Design review of the part built by this model. Coordinates are the model's own, in mm. Give positions to 0.01 mm unless a question says otherwise; leave off trailing zeros. Write each loop counter-clockwise with the first axis right and the second up, starting at its lowest first coordinate (ties: lowest second). Pieces come first, ordered by that corner, then holes. Notation, with made-up numbers: (12.25, 34.25) -> (51.25, 34.25) arc R23 ccw to (51.25, 60.25) -> close; hole circle Ø9 at (14, 27). An arc over 180 degrees is marked (long way). Use CSV: the item, a comma, the result in double quotes.
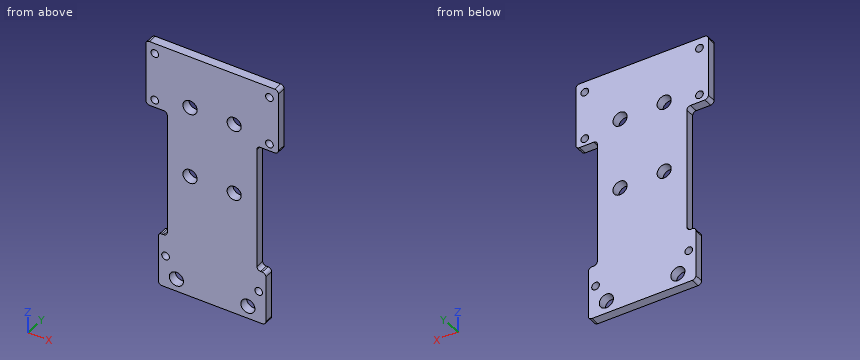
Autodesk Inventor part; units mm, degrees
ref_plane "YZ Plane" through (0, 0, 0) normal (1, 0, 0) x (0, 1, 0)
ref_plane "XZ Plane" through (0, 0, 0) normal (0, 1, 0) x (-1, 0, 0)
ref_plane "XY Plane" through (0, 0, 0) normal (0, 0, 1) x (1, 0, 0)
sketch "Sketch2" plane through (0, 0, 0) normal (0, 1, 0) x (-1, 0, 0)
  line L0 (35, 0) -> (-35, 0)
  line L1 (-37, -2) -> (-37, -35)
  line L2 (-35, -37) -> (-27, -37)
  line L3 (-25, -39) -> (-25, -107)
  line L4 (-27, -109) -> (-28, -109)
  line L5 (-30, -111) -> (-30, -137)
  line L6 (-28, -139) -> (28, -139)
  line L7 (30, -137) -> (30, -111)
  line L8 (28, -109) -> (27, -109)
  line L9 (25, -107) -> (25, -39)
  line L10 (27, -37) -> (35, -37)
  line L11 (37, -35) -> (37, -2)
  circle A0 centre (19.95, -132) radius 3.95
  circle A1 centre (-19.95, -132) radius 3.95
  circle A2 centre (26, -121) radius 2.15
  circle A3 centre (-26, -121) radius 2.15
  circle A4 centre (12.319, -69.4) radius 3.95
  circle A5 centre (-12.321, -69.4) radius 3.95
  circle A6 centre (12.319, -29.4) radius 3.95
  circle A7 centre (-12.319, -29.4) radius 3.95
  circle A8 centre (32, -32.8) radius 2.15
  circle A9 centre (32, -5.8) radius 2.15
  circle A10 centre (-32, -33) radius 2.15
  circle A11 centre (-32, -6) radius 2.15
  arc A12 (25, -107) -> (27, -109) centre (27, -107) ccw
  arc A13 (30, -111) -> (28, -109) centre (28, -111) ccw
  arc A14 (27, -37) -> (25, -39) centre (27, -39) ccw
  arc A15 (35, -37) -> (37, -35) centre (35, -35) ccw
  arc A16 (37, -2) -> (35, 0) centre (35, -2) ccw
  arc A17 (-35, 0) -> (-37, -2) centre (-35, -2) ccw
  arc A18 (-37, -35) -> (-35, -37) centre (-35, -35) ccw
  arc A19 (-25, -39) -> (-27, -37) centre (-27, -39) ccw
  arc A20 (-27, -109) -> (-25, -107) centre (-27, -107) ccw
  arc A21 (-28, -109) -> (-30, -111) centre (-28, -111) ccw
  arc A22 (-30, -137) -> (-28, -139) centre (-28, -137) ccw
  arc A23 (28, -139) -> (30, -137) centre (28, -137) ccw
  point P0 (0, 0)
  point P1 (37, 0)
  point P2 (-37, 0)
  point P3 (-37, -37)
  point P4 (-25, -37)
  point P5 (-25, -109)
  point P6 (-30, -109)
  point P7 (-30, -139)
  point P8 (30, -139)
  point P9 (30, -109)
  point P10 (25, -109)
  point P11 (25, -37)
  point P12 (37, -37)
  dimension "d71" = 74
  dimension "d72" = 37
  dimension "d73" = 12
  dimension "d74" = 72
  dimension "d76" = 30
  dimension "d77" = 60
  dimension "d78" = 30
  dimension "d79" = 5
  dimension "d80" = 72
  dimension "d81" = 12
  dimension "d82" = 7.9
  dimension "d83" = 7.9
  dimension "d84" = 39.9
  dimension "d85" = 7
  dimension "d86" = 7
  dimension "d87" = 37
  dimension "d88" = 4.3
  dimension "d89" = 11
  dimension "d90" = 4
  dimension "d91" = 4.3
  dimension "d92" = 5
  dimension "d93" = 11
  dimension "d94" = 4
  dimension "d95" = 52
  dimension "d96" = 7.9
  dimension "d97" = 7.9
  dimension "d98" = 7.9
  dimension "d99" = 7.9
  dimension "d100" = 24.64
  dimension "d101" = 24.638
  dimension "d102" = 12.319
  dimension "d103" = 12.319
  dimension "d104" = 40
  dimension "d105" = 29.4
  dimension "d108" = 19.95
  dimension "d109" = 4.3
  dimension "d110" = 4.3
  dimension "d111" = 4.3
  dimension "d112" = 4.3
  dimension "d113" = 27
  dimension "d114" = 27
  dimension "d115" = 5
  dimension "d116" = 5
  dimension "d117" = 6
  dimension "d118" = 5.8
  dimension "d121" = 37
  dimension "d122" = 2
  dimension "d123" = 5
  dimension "d124" = 5
  dimension "d125" = 30
extrude "Extrusion3" add sketch "Sketch2" along normal blind 5
properties part number "BottomSupport"
(1) Take a section at D-D (y = 1.7). State how many separate pieces and enclosed holes the cut face has, then the cut area to 3 significant figures.
Established:
separate pieces,"1"
enclosed holes,"12"
area,"7,750 mm2"
(2) Clearance check with flat-ended pins moving along their axes: pin 1 (7 mm diameter, centred on x = -12.319, z = -29.4, fed in from +Y); pin 2 (1 mm diameter, centred on x = 0.5, y = 1, fed in from +Z); pin 3 (1.5 mm diameter, centred on x = 29.5, y = 3, fed in from -Z); pin 4 (1 mm diameter, centred on y = 2.5, z = -70.5, fed in from -X). State where each tip first meets the part, or that it passes through.
Established:
pin 1,"passes through"
pin 2,"stops at z = 0"
pin 3,"stops at z = -138.85"
pin 4,"stops at x = -25"
(3) For line 1 along Z through (x, y) = (32, 2.1); line 2 along Z through (x, y) = (12, 0.25); line 3 along Z through (x, y) = (-20, 2.15), list the stretches that pass through material, from the lowest coordinate up. Write a range as [from, to].
Established:
line 1,"z = [-37, -35.15], [-30.85, -8.15], [-3.85, 0]"
line 2,"z = [-139, -73.34], [-65.46, -33.34], [-25.46, 0]"
line 3,"z = [-139, -135.95], [-128.05, 0]"
(4) Take a section at A-A (z = -121). Write out the cut boundary in (x, y), then the cut area to 3 significant figures.
Established:
outline,"(-30, 0) -> (-28.15, 0) -> (-28.15, 5) -> (-30, 5) -> close; (-23.85, 0) -> (23.85, 0) -> (23.85, 5) -> (-23.85, 5) -> close; (28.15, 0) -> (30, 0) -> (30, 5) -> (28.15, 5) -> close"
area,"257 mm2"
(5) Take a section at C-C (x = -19.95). Write out the cut boundary in (y, z), then the cut area to 4 significant figures.
Established:
outline,"(0, -139) -> (5, -139) -> (5, -135.95) -> (0, -135.95) -> close; (0, -128.05) -> (5, -128.05) -> (5, 0) -> (0, 0) -> close"
area,"655.5 mm2"
(6) Take a section at B-B (x = 32). Write out the cut boundary in (y, z).
Established:
outline,"(0, -37) -> (5, -37) -> (5, -35.15) -> (0, -35.15) -> close; (0, -30.85) -> (5, -30.85) -> (5, -8.15) -> (0, -8.15) -> close; (0, -3.85) -> (5, -3.85) -> (5, 0) -> (0, 0) -> close"
